Geometry check sheet. Reference: the model listing, model coordinates, mm. A direction names the side the tool comes from. Give positions to 0.01 mm unless a question says otherwise; leave off trailing zeros. Loops run counter-clockwise (first coordinate to the right, second up) from the corner with the lowest first, then second, coordinate; pieces in that order, holes last. Notation, with made-up numbers: (54, -30) - (98, -30) arc R10 ccw to (98, -11) - close; hole circle Ø2 at (-17, -36.5). An arc over 180 degrees is marked (long way). Use a Markdown table: item, result. Add a question column.
1. Set-up check for faces 5 (the flat face through (109, 20.794, 2)), 6 (the flat face through (39.809, 8.085, 1.726)), 7 (the flat face through (40.94, -8.03, 1.73)): record each of +Z, -Z, +X, -X, +Y, -Y from which the full face is reachable in a straight line by a thin tool's end or side.
2. Draft check along Y on faces 1 (the cylindrical face through (82.59, -6.64, 1.77)), 2 (the cylindrical face through (-10, 0, 2)), 3 (the flat face through (50, 0, 0)), 4 (the flat face through (109, -20.794, 2)). Enter one of: pulls with the +Y half, pulls with the -Y half, needs draft (parallel to the pull), parting line crosses it, or undercut.
3. Material ranges on L1, parallel to Y at x = 0, z = 1.1; L2, parallel to X at y = -1, z = 1.5; L3, parallel to Y at x = 66.5, z = 2.55, recorded low to high.
4. Depth check by flat-ended pin: P1, Ø3, axis at x = 0, y = 0, coming from the -Z side; P2, Ø1.5, axis at x = 60, z = 1.5, coming from the +Y side. Enter the tip coordinate at first touch or a pass-through.
5. Cross-section at A-A on z = 2.75. Enter the section's corners in (x, y), and give its area (3 significant figures).
6. Cross-section at C-C on x = 78.5. Enter the section's corners in (y, z), and give its area (3 significant figures).
7. Cross-section at B-B on y = -18. Enter the section's corners in (x, z).
from build123d import *

# Parameters (mm, degrees)
EXTRUSION1_DEPTH = 3.5
CONG_1_R         = 3
CONG_2_R         = 3
CONG_3_R         = 1
CONG_4_R         = 1
CONG_7_R         = 0.2
CONG_8_R         = 0.2
ESQUISSE2_R      = 2
EXTRUSION2_DEPTH = 3.5


with BuildPart() as part:
    # Esquisse1 → Extrusion1 (new body)
    with BuildSketch(Plane.XY):
        with BuildLine():
            Line((0, 10), (83.162526199, 6))
            ThreePointArc((83.162526199, 6), (92.806251136, 21.462176031), (110, 27.5))
            Line((110, 27.5), (110, 20.794494718))
            Line((110, 20.794494718), (108, 20.794494718))
            Line((108, 20.794494718), (108, 21.9089023))
            ThreePointArc((108, 21.9089023), (88, 0), (108, -21.9089023))
            Line((108, -21.9089023), (108, -20.794494718))
            Line((108, -20.794494718), (110, -20.794494718))
            Line((110, -20.794494718), (110, -27.5))
            ThreePointArc((110, -27.5), (92.806251136, -21.462176031), (83.162526199, -6))
            Line((83.162526199, -6), (0, -10))
            ThreePointArc((0, -10), (-10, 0), (0, 10))
        make_face()
    extrude(amount=EXTRUSION1_DEPTH)

    # Congé1
    cong_1_edges = [part.edges().sort_by_distance(p)[0] for p in [
        (83.162526199, 6, 1.75),
    ]]
    fillet(cong_1_edges, radius=CONG_1_R)

    # Congé2
    cong_2_edges = [part.edges().sort_by_distance(p)[0] for p in [
        (83.162526199, -6, 1.75),
    ]]
    fillet(cong_2_edges, radius=CONG_2_R)

    # Congé3
    cong_3_edges = [part.edges().sort_by_distance(p)[0] for p in [
        (110, 27.5, 1.75),
    ]]
    fillet(cong_3_edges, radius=CONG_3_R)

    # Congé4
    cong_4_edges = [part.edges().sort_by_distance(p)[0] for p in [
        (110, -27.5, 1.75),
    ]]
    fillet(cong_4_edges, radius=CONG_4_R)

    # Congé7
    cong_7_edges = [part.edges().sort_by_distance(p)[0] for p in [
        (108, -21.9089023, 1.75),
    ]]
    fillet(cong_7_edges, radius=CONG_7_R)

    # Congé8
    cong_8_edges = [part.edges().sort_by_distance(p)[0] for p in [
        (108, 21.9089023, 1.75),
    ]]
    fillet(cong_8_edges, radius=CONG_8_R)

    # Esquisse2 → Extrusion2 (cut)
    with BuildSketch(Plane.XY.offset(3.5)):
        Circle(ESQUISSE2_R)
    extrude(amount=-EXTRUSION2_DEPTH, mode=Mode.SUBTRACT)


solid = part.part
Values found:
| question | item | result |
|---|---|---|
| 1 | face 5 | +Z, -Z, +X |
| 1 | face 6 | +Z, -Z, +Y |
| 1 | face 7 | +Z, -Z, -Y |
| 2 | face 1 | pulls with the -Y half |
| 2 | face 2 | parting line crosses it |
| 2 | face 3 | needs draft |
| 2 | face 4 | undercut |
| 3 | L1 | y = -10 to -2, 2 to 10 |
| 3 | L2 | x = -9.95 to -1.73, 1.73 to 88.02 |
| 3 | L3 | y = -6.8 to 6.8 |
| 4 | P1 | passes through |
| 4 | P2 | stops at y = 7.15 |
| 5 | outline | (0, -10) - (80.75, -6.12) arc R3 cw to (83.76, -8.22) arc R27.5 ccw to (108.96, -27.48) arc R1 ccw to (110, -26.48) - (110, -20.79) - (108, -20.79) - (108, -21.69) arc R0.2 cw to (107.78, -21.89) arc R22 cw to (107.78, 21.89) arc R0.2 cw to (108, 21.69) - (108, 20.79) - (110, 20.79) - (110, 26.48) arc R1 ccw to (108.96, 27.48) arc R27.5 ccw to (83.76, 8.22) arc R3 cw to (80.75, 6.12) - (0, 10) arc R10 ccw to start; hole circle Ø4 at (0, 0) |
| 5 | area | 1,900 mm2 |
| 6 | outline | (-6.22, 0) - (6.22, 0) - (6.22, 3.5) - (-6.22, 3.5) - close |
| 6 | area | 43.6 mm2 |
| 7 | outline | (89.21, 0) - (97.35, 0) - (97.35, 3.5) - (89.21, 3.5) - close |
